Source: three-view drawing plus pictorial views. Frame: mm from the lowest corner of the part. A direction names the side the tool comes from. Round coordinates to 2 decimals unless told otherwise and drop trailing zeros. Write each loop counter-clockwise with the first axis right and the second up, starting at its lowest first coordinate (ties: lowest second). Pieces come first, ordered by that corner, then holes. Notation, with made-up numbers: M 26,-29.5 L 38,-29.5 A25 cw 38,-15.5 Z; hole C -37,61 d6. An arc over 180 degrees is marked long. Answer as CSV lines item,"result". Start each with the question number.
Q1. First-contact query: pin 1 (1.5 mm diameter, centred on x = 4.5, z = 14.5, fed in from +Y); pin 2 (1.2 mm diameter, centred on x = 8, y = 22, fed in from +Z); pin 3 (10 mm diameter, centred on y = 27, z = 15, fed in from -X); pin 4 (5 mm diameter, centred on x = 6.5, z = 6, fed in from +Y). Flat tips, straight axial feed; report the tip coordinate or a pass-through.
Q2. Reachability of the marked faces 1, 2, 3, 4 and 5 from +Z, -Z, +X, -X, +Y, -Y: full face, straight path, thin tool, end or side. Return the list, or none.
Q3. Section query A-A on x = 4. Output: boundary loops of the cut face in (y, z).
Q4. Section query C-C on z = 10. Output: boundary loops of the cut face in (x, y), and give its area (3 significant figures).
Q5. Section query D-D on x = 10.75. Output: boundary loops of the cut face in (y, z), and give its area (3 significant figures).
Q6. Section query B-B on y = 28. Output: boundary loops of the cut face in (x, z), and give its area (3 significant figures).
Q7. Ray query, probe 1 along Y at (x, z) = (11.5, 28.5); probe 2 along Y at (x, z) = (10.75, 5.5); probe 3 along Z at (x, y) = (3.25, 8.75). Return the intervals inside material, ascending.
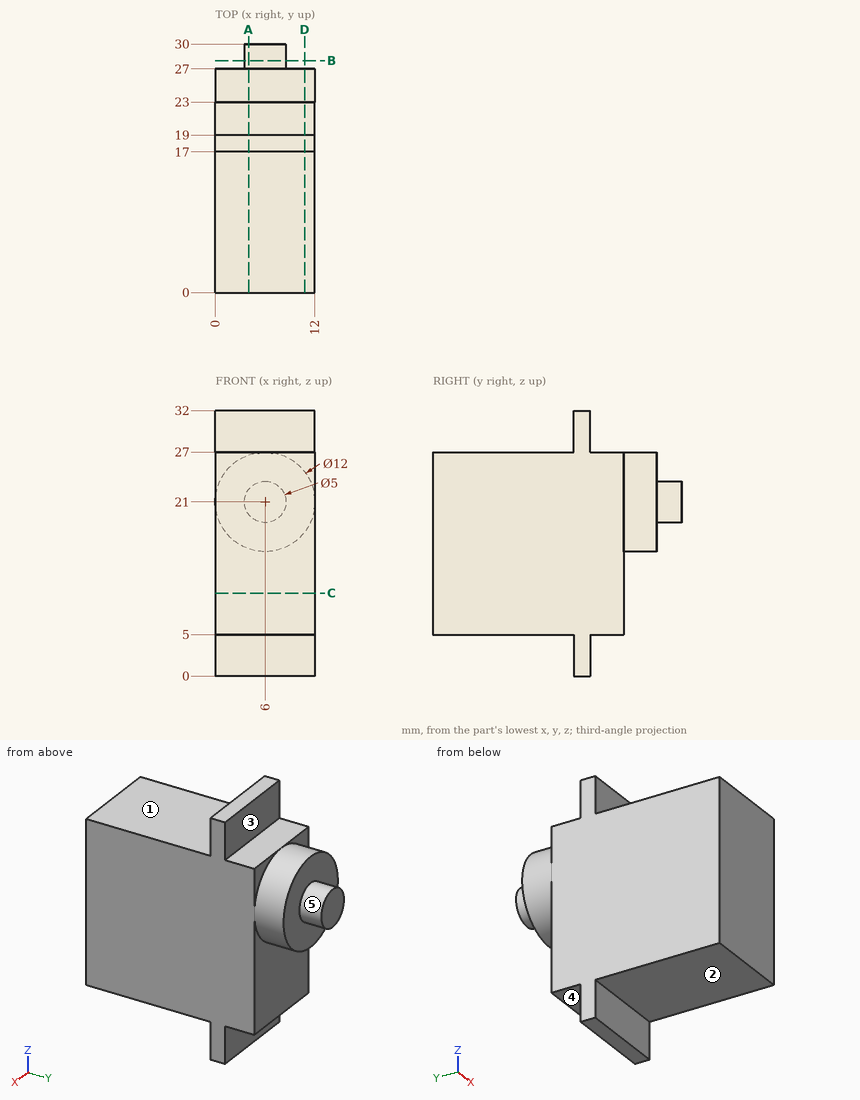
Entries:
1,pin 1,"stops at y = 27"
1,pin 2,"stops at z = 27"
1,pin 3,"stops at x = 0"
1,pin 4,"stops at y = 23"
2,face 1,"+Z, +X, -X, -Y"
2,face 2,"-Z, +X, -X, -Y"
2,face 3,"+Z, +X, -X, +Y"
2,face 4,"-Z, +X, -X, +Y"
2,face 5,"+Y"
3,outline,"M 0,5 L 17,5 L 17,0 L 19,0 L 19,5 L 23,5 L 23,15.34 L 27,15.34 L 27,19.5 L 30,19.5 L 30,22.5 L 27,22.5 L 27,26.66 L 23,26.66 L 23,27 L 19,27 L 19,32 L 17,32 L 17,27 L 0,27 Z"
4,outline,"M 0,0 L 12,0 L 12,23 L 0,23 Z"
4,area,"276 mm^2"
5,outline,"M 0,5 L 17,5 L 17,0 L 19,0 L 19,5 L 23,5 L 23,17.33 L 27,17.33 L 27,24.67 L 23,24.67 L 23,27 L 19,27 L 19,32 L 17,32 L 17,27 L 0,27 Z"
5,area,"555 mm^2"
6,outline,"C 6,21 d5"
6,area,"19.6 mm^2"
7,probe 1,"y = 17 to 19"
7,probe 2,"y = 0 to 23"
7,probe 3,"z = 5 to 27"
